```python
from build123d import *


with BuildPart() as part:
    # Croquis1 → Revolución1 (revolve)
    with BuildSketch(Plane(origin=(0, 0, 0), x_dir=(0, 0, -1), z_dir=(1, 0, 0))):
        with BuildLine():
            Line((-40, 0), (40, 0))
            Line((40, 0), (40, -40))
            Line((40, -40), (35, -44))
            Line((35, -44), (35, -52))
            Line((35, -52), (40, -56))
            Line((40, -56), (40, -72.044897428))
            ThreePointArc((40, -72.044897428), (15, -82.55), (-10, -72.044897428))
            Line((-10, -72.044897428), (-10, -56))
            Line((-10, -56), (-5, -52))
            Line((-5, -52), (-5, -44))
            Line((-5, -44), (-10, -40))
            Line((-10, -40), (-10, -5))
            Line((-10, -5), (-40, -5))
            Line((-40, -5), (-40, 0))
        make_face()
    revolve(axis=Axis((0, 0, 40), (0, 0, -1)))


solid = part.part
```
Work out the finished part from the listing and answer in its coordinate system (mm). A direction names the side the tool comes from. Coordinates: 2 decimals unless noted, no trailing zeros. Loops run counter-clockwise (first coordinate to the right, second up) from the corner with the lowest first, then second, coordinate; pieces in that order, holes last. Notation, with made-up numbers: (89.25, -26) - (127.25, -26) arc R31 cw to (127.25, 2) - close; hole circle Ø7 at (80.25, 16). An arc over 180 degrees is marked (long way). Use a Markdown table: item, result.
Item 1: Find section D-D, the plane z = -4.5. Determine the outline of the cut face in (x, y), and give its area (3 significant figures).
Evaluation:
| item | result |
|---|---|
| outline | circle Ø161.88 at (0, 0) |
| area | 20,600 mm2 |
Item 2: Consider probe 1 along Z at (x, y) = (-15, -30); probe 2 along Y at (x, z) = (-1, 8); probe 3 along Z at (x, y) = (-39, -32). Determine where each line is inside the solid, lowest interval first. Write a range as from..to.
Evaluation:
| item | result |
|---|---|
| probe 1 | z = -40..10 |
| probe 2 | y = -73.93..-54.39, -41.59..41.59, 54.39..73.93 |
| probe 3 | z = -35..5 |
Item 3: For faces 1 (the flat face through (-12, -43, -35)), 2 (the flat face through (42.4, 37, -40)), 3 (the flat face through (-12, 43, 5)), determine the directions among +Z, -Z, +X, -X, +Y, -Y from which every point of the face is accessible in a straight line to the end or side of a thin tool.
Evaluation:
| item | result |
|---|---|
| face 1 | -Z |
| face 2 | -Z, +X, -X, +Y, -Y |
| face 3 | +Z |
Item 4: Find section C-C, the plane z = 21.5. Determine the outline of the cut face in (x, y).
Evaluation:
| item | result |
|---|---|
| outline | circle Ø10 at (0, 0) |
Item 5: Given pin 1 Ø6 at (x, y) = (32.5, -27) entering from -Z; pin 2 Ø6 at (x, y) = (52, -5) entering from -Z; pin 3 Ø2 at (x, y) = (-22, -31.5) entering from +Z; pin 4 Ø10 at (y, z) = (27.5, 4.5) entering from +X, each flat-ended and moving along its own axis, determine where each tip first touches the part or whether it passes through.
Evaluation:
| item | result |
|---|---|
| pin 1 | stops at z = -40 |
| pin 2 | stops at z = -39.05 |
| pin 3 | stops at z = 10 |
| pin 4 | stops at x = 75.04 |
Item 6: Find section A-A, the plane y = 0. Determine the outline of the cut face in (x, z), and give its area (3 significant figures).
Evaluation:
| item | result |
|---|---|
| outline | (-72.04, -40) - (-56, -40) - (-52, -35) - (-44, -35) - (-40, -40) - (40, -40) - (44, -35) - (52, -35) - (56, -40) - (72.04, -40) arc R35 ccw to (72.04, 10) - (56, 10) - (52, 5) - (44, 5) - (40, 10) - (5, 10) - (5, 40) - (-5, 40) - (-5, 10) - (-40, 10) - (-44, 5) - (-52, 5) - (-56, 10) - (-72.04, 10) arc R35 ccw to start |
| area | 7,990 mm2 |
Item 7: The mould has two halves that part along Y. Classify faces 4 (the flat face through (42.4, -37, 10)), 5 (the cylindrical face through (4.88, 1.08, 25.21)), 6 (the conical face through (-15.68, -49.78, 5.24)): +Y half, -Y half, draft (parallel to the pull), parting line (faces both ways), or undercut.
Evaluation:
| item | result |
|---|---|
| face 4 | draft |
| face 5 | parting line |
| face 6 | undercut |
